Geometry: final body of the model. Coordinates: model frame, mm. Face numbers are marked on the shaded views. Coordinates: 2 decimals unless noted, no trailing zeros. Order: outer loops, then holes, each group sorted by start corner. A loop starts at its lowest first (then second) coordinate and runs counter-clockwise, first axis right, second up. Notation, with made-up numbers: M 22,47.5 L 76,47.5 A14 cw 76,59.5 Z; hole C 3,14 d8. An arc over 180 degrees is marked long. One line per question, with ' | ' between items.
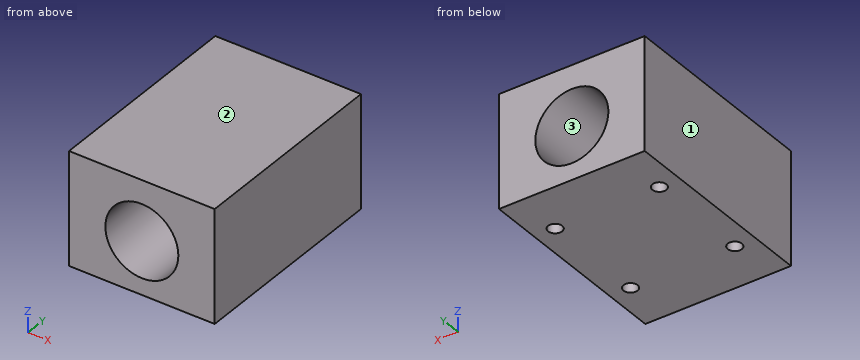
from build123d import *

# Parameters (mm, degrees)
SKETCH1_W                  = 41.91
SKETCH1_H                  = 32.5
BOSS_EXTRUDE1_DEPTH        = 59.1185
SKETCH2_R                  = 10.5
CUT_EXTRUDE1_DEPTH         = 60.1185
F_10_32_TAPPED_HOLE1_D     = 4.0386
F_10_32_TAPPED_HOLE1_DEPTH = 9.906
F_10_32_TAPPED_HOLE1_TIP   = 1.213317848


with BuildPart() as part:
    # Sketch1 → Boss-Extrude1 (new body)
    with BuildSketch(Plane(origin=(0, 0, 0), x_dir=(1, 0, 0), z_dir=(0, 1, 0))):
        Rectangle(SKETCH1_W, SKETCH1_H)
    extrude(amount=BOSS_EXTRUDE1_DEPTH)

    # Sketch2 → Cut-Extrude1 (cut, through all)
    with BuildSketch(Plane(origin=(0, 59.1185, 0), x_dir=(1, 0, 0), z_dir=(0, 1, 0))):
        with Locations((0, 1.01)):
            Circle(SKETCH2_R)
    extrude(amount=-CUT_EXTRUDE1_DEPTH, mode=Mode.SUBTRACT)

    # #10-32 Tapped Hole1
    with Locations(Plane(origin=(0, 0, -16.25), x_dir=(-1, 0, 0), z_dir=(0, 0, -1))):
        with Locations((-14.986, 14.31925), (14.986, 14.31925), (14.986, 44.79925), (-14.986, 44.79925)):
            Hole(F_10_32_TAPPED_HOLE1_D / 2, depth=F_10_32_TAPPED_HOLE1_DEPTH)
            with Locations((0, 0, -(F_10_32_TAPPED_HOLE1_DEPTH + F_10_32_TAPPED_HOLE1_TIP / 2))):  # 118° drill point
                Cone(0, F_10_32_TAPPED_HOLE1_D / 2, F_10_32_TAPPED_HOLE1_TIP, mode=Mode.SUBTRACT)


solid = part.part
1. Pin query (flat end, axial travel): P1, Ø3.5, axis at x = 14.99, y = 44.8, coming from the -Z side. Return the tip coordinate at first contact, or that it passes through.
Response values:
P1: stops at z = -6.18
2. Material intervals for line 1 (Z direction, x = 0, y = 32); line 2 (X direction, y = 37, z = -1.01) (3 decimals); line 3 (X direction, y = 26, z = 5) (3 decimals), sorted ascending. Write a range as [from, to].
Response values:
line 1: z = [-16.25, -11.51], [9.49, 16.25] | line 2: x = [-20.955, -10.5], [10.5, 20.955] | line 3: x = [-20.955, -8.61], [8.61, 20.955]
3. Section A-A, the plane x = 0. Output: boundary loops of the cut face in (y, z), and give its area (3 significant figures).
Response values:
outline: M 0,-16.25 L 59.12,-16.25 L 59.12,-11.51 L 0,-11.51 Z; M 0,9.49 L 59.12,9.49 L 59.12,16.25 L 0,16.25 Z | area: 680 mm^2
4. Draft query along Z for the marked faces 1, 2 and 3. Return one class per face: pulls with the +Z half, pulls with the -Z half, needs draft (parallel to the pull), parting line crosses it, or undercut.
Response values:
face 1: needs draft | face 2: pulls with the +Z half | face 3: undercut
5. Section B-B, the plane z = -1.01. Output: boundary loops of the cut face in (x, y) (1 decimal).
Response values:
outline: M -21,0 L -10.5,0 L -10.5,59.1 L -21,59.1 Z; M 10.5,0 L 21,0 L 21,59.1 L 10.5,59.1 Z
6. Section C-C, the plane y = 18.5. Output: boundary loops of the cut face in (x, z) (3 decimals), and give its area (3 significant figures).
Response values:
outline: M -20.955,-16.25 L 20.955,-16.25 L 20.955,16.25 L -20.955,16.25 Z; hole C 0,-1.01 d21 | area: 1,020 mm^2
7. Section D-D, the plane z = -8. Output: boundary loops of the cut face in (x, y) (1 decimal).
Response values:
outline: M -21,0 L -7.8,0 L -7.8,59.1 L -21,59.1 Z; M 7.8,0 L 21,0 L 21,59.1 L 7.8,59.1 Z; hole C -15,14.3 d4; hole C -15,44.8 d4; hole C 15,14.3 d4; hole C 15,44.8 d4
